For this review, take the finished solid that the model builds, in its own axes (mm). A direction names the side the tool comes from. Give positions to 0.01 mm unless a question says otherwise; leave off trailing zeros. Loops run counter-clockwise (first coordinate to the right, second up) from the corner with the lowest first, then second, coordinate; pieces in that order, holes last. Notation, with made-up numbers: (23.5, 67) - (63.5, 67) arc R16 cw to (63.5, 76) - close; hole circle Ø9 at (1.5, 4). An arc over 180 degrees is marked (long way). Use CSV: the item, a comma, the result in double quotes. Start each with the question number.
1. For faces 5 (the flat face through (-26, 53, 5)), 6 (the cylindrical face through (-32.24, 68.73, 2.46)), list the 3-axis set-ups (+Z, -Z, +X, -X, +Y, -Y) from which the entire face can be reached by the end or side of a thin tool; tool diameter is ignored.
2. Take a section at B-B on x = 7. Give the boundary of the cut face in (y, z).
3. Take a section at A-A on y = 55. Give the boundary of the cut face in (x, z), plus the area to 3 significant figures.
4. For pin 1 (2 mm diameter, centred on x = -42.5, z = 1, fed in from -Y); pin 2 (12 mm diameter, centred on x = -26.5, y = 59, fed in from +Z); pin 3 (2 mm diameter, centred on y = 11.5, z = 4.5, fed in from -X), all flat-tipped, find the tip position at first contact; note any pin that passes through.
5. Mouldability with a two-part tool opening along X and no side actions: class faces 1 (the flat face through (-36.1, 6.13, 2.46)), 2 (the cylindrical face through (22, 40, 2)), 3 (the cylindrical face through (-1.319, 99.985, 2.465)), 4 (the flat face through (-26, 53, 0)) as pulls with the +X half, pulls with the -X half, needs draft (parallel to the pull), parting line crosses it, or undercut.
6. Take a section at C-C on z = 1.5. Give the boundary of the cut face in (x, y), plus the area to 3 significant figures.
7. Wall thickness on line 1 (X direction, y = 44, z = 0.75); line 2 (X direction, y = 85, z = 2.75); line 3 (Y direction, x = -32.5, z = 3.3): over which ranges is each line inside the solid? List them lowest first.
```python
from build123d import *

# Parameters (mm, degrees)
SZKIC1_R                    = 10.5
DODANIE_WYCI_GNI_CIE1_DEPTH = 5


with BuildPart() as part:
    # Szkic1 → Dodanie-wyciągnięcie1 (new body)
    with BuildSketch(Plane.XY):
        with BuildLine():
            Line((-17.23880927, -15.225749734), (-55.491242037, 28.084195861))
            ThreePointArc((-55.491242037, 28.084195861), (-58.835117414, 33.629849165), (-60, 40))
            ThreePointArc((-60, 40), (0, 100), (60, 40))
            ThreePointArc((60, 40), (58.835117414, 33.629849165), (55.491242037, 28.084195861))
            Line((55.491242037, 28.084195861), (17.23880927, -15.225749734))
            ThreePointArc((17.23880927, -15.225749734), (0, -23), (-17.23880927, -15.225749734))
        make_face()
        with Locations((-32.5, 40)):
            Circle(SZKIC1_R, mode=Mode.SUBTRACT)
        with Locations((32.5, 40)):
            Circle(SZKIC1_R, mode=Mode.SUBTRACT)
        with BuildLine():
            Line((-23.232277997, 8.17672768), (-8.994161358, -7.943869426))
            ThreePointArc((-8.994161358, -7.943869426), (0, -12), (8.994161358, -7.943869426))
            Line((8.994161358, -7.943869426), (23.232277997, 8.17672768))
            ThreePointArc((23.232277997, 8.17672768), (26.972823751, 18.81529275), (22.24478815, 29.053282232))
            ThreePointArc((22.24478815, 29.053282232), (17.552836173, 41.257892492), (24.218531469, 52.506689369))
            ThreePointArc((24.218531469, 52.506689369), (32.255432897, 68.469423949), (22.572828784, 83.491003675))
            ThreePointArc((22.572828784, 83.491003675), (0, 89), (-22.572828784, 83.491003675))
            ThreePointArc((-22.572828784, 83.491003675), (-32.255432897, 68.469423949), (-24.218531469, 52.506689369))
            ThreePointArc((-24.218531469, 52.506689369), (-17.552836173, 41.257892492), (-22.24478815, 29.053282232))
            ThreePointArc((-22.24478815, 29.053282232), (-26.972823751, 18.81529275), (-23.232277997, 8.17672768))
        make_face(mode=Mode.SUBTRACT)
    extrude(amount=DODANIE_WYCI_GNI_CIE1_DEPTH)


solid = part.part
```
Check result:
1,face 5,"+Z, +X, -X, +Y, -Y"
1,face 6,"+Z, -Z"
2,outline,"(-21.91, 0) - (-9.75, 0) - (-9.75, 5) - (-21.91, 5) - close; (88.5, 0) - (99.59, 0) - (99.59, 5) - (88.5, 5) - close"
3,outline,"(-58.09, 0) - (-27.22, 0) - (-27.22, 5) - (-58.09, 5) - close; (27.22, 0) - (58.09, 0) - (58.09, 5) - (27.22, 5) - close"
3,area,"309 mm²"
4,pin 1,"stops at y = 12.24"
4,pin 2,"stops at z = 5"
4,pin 3,"stops at x = -41.73"
5,face 1,"pulls with the -X half"
5,face 2,"undercut"
5,face 3,"parting line crosses it"
5,face 4,"needs draft"
6,outline,"(-60, 40) arc R18 ccw to (-55.49, 28.08) - (-17.24, -15.23) arc R23 ccw to (17.24, -15.23) - (55.49, 28.08) arc R18 ccw to (60, 40) arc R60 ccw to start; hole circle Ø21 at (-32.5, 40); hole (-24.22, 52.51) arc R15 cw to (-22.24, 29.05) arc R15 ccw to (-23.23, 8.18) - (-8.99, -7.94) arc R12 ccw to (8.99, -7.94) - (23.23, 8.18) arc R15 ccw to (22.24, 29.05) arc R15 cw to (24.22, 52.51) arc R18 ccw to (22.57, 83.49) arc R49 ccw to (-22.57, 83.49) arc R18 ccw to start; hole circle Ø21 at (32.5, 40)"
6,area,"5,140 mm²"
7,line 1,"x = -59.87 to -42.21, -22.79 to -18.04, 18.04 to 22.79, 42.21 to 59.87"
7,line 2,"x = -39.69 to -19.39, 19.39 to 39.69"
7,line 3,"y = 2.05 to 29.5, 50.5 to 90.44"
